Could you check a few things on this model? Use its own coordinates, in mm. A direction names the side the tool comes from. Give positions to 0.01 mm unless a question says otherwise; leave off trailing zeros. Loops run counter-clockwise (first coordinate to the right, second up) from the corner with the lowest first, then second, coordinate; pieces in that order, holes last.
1. Imagine slicing it at C-C (z = 113.65). List the corners of the cut face in (x, y) for me.
2. Thinking about a two-plate mould opening in X: for faces 3 (the cylindrical face through (42.64, 1.48, 36.93)), 4 (the flat face through (43, 1, 127)), 5 (the cylindrical face through (87.1, 1.52, 0.86)), which applies, +X half, -X half, draft (parallel to the pull), parting line (faces both ways), or undercut?
3. For faces 1 (the flat face through (43, 1, 0)), 2 (the cylindrical face through (6.03, 1.48, 48.25)), which set-ups out of +Z, -Z, +X, -X, +Y, -Y let a thin tool reach every point of the face, with its end or its side?
4. Imagine slicing it at A-A (z = 33.65). Count the separate pieces of the cut face and the enclosed holes in it, plus the area to 3 significant figures.
5. For P1, Ø4, axis at x = 44, z = 93.5, coming from the -Y side, with a flat end and sliding along its axis, tell me the tip position at first contact or that it passes through.
6. I need wall thicknesses on line 1 along X through (y, z) = (2.4, 86.5); line 2 along X through (y, z) = (0.3, 41); line 3 along X through (y, z) = (1.7, 50.5). Which ranges of each line are inside material? Lowest first, please.
7. Imagine slicing it at B-B (x = 6). List the corners of the cut face in (y, z) for me.
```python
from build123d import *

# Parameters (mm, degrees)
SKETCH_1_W      = 88
SKETCH_1_H      = 127
SKETCH_1_R      = 3.55
SKETCH_1_R_2    = 2.55
EXTRUDE_1_DEPTH = 3
FILLET_1_R      = 3


with BuildPart() as part:
    # 草图1 → 凸台-拉伸1 (new body)
    with BuildSketch(Plane(origin=(0, 0, 0), x_dir=(1, 0, 0), z_dir=(0, 1, 0))):
        with Locations((44, -63.5)):
            Rectangle(SKETCH_1_W, SKETCH_1_H)
        with Locations(Location((13.68, -13.65, 0), (0, 0, 270))):
            Circle(SKETCH_1_R, mode=Mode.SUBTRACT)
        with Locations(Location((44, -13.65, 0), (0, 0, 270))):
            Circle(SKETCH_1_R, mode=Mode.SUBTRACT)
        with Locations(Location((74.32, -13.65, 0), (0, 0, 270))):
            Circle(SKETCH_1_R, mode=Mode.SUBTRACT)
        with Locations(Location((44, -23.65, 0), (0, 0, 270))):
            Circle(SKETCH_1_R, mode=Mode.SUBTRACT)
        with Locations(Location((74.32, -23.65, 0), (0, 0, 270))):
            Circle(SKETCH_1_R, mode=Mode.SUBTRACT)
        with Locations(Location((44, -33.65, 0), (0, 0, 270))):
            Circle(SKETCH_1_R, mode=Mode.SUBTRACT)
        with Locations(Location((74.32, -33.65, 0), (0, 0, 270))):
            Circle(SKETCH_1_R, mode=Mode.SUBTRACT)
        with Locations(Location((44, -43.65, 0), (0, 0, 270))):
            Circle(SKETCH_1_R, mode=Mode.SUBTRACT)
        with Locations(Location((74.32, -43.65, 0), (0, 0, 270))):
            Circle(SKETCH_1_R, mode=Mode.SUBTRACT)
        with Locations(Location((13.68, -23.65, 0), (0, 0, 270))):
            Circle(SKETCH_1_R, mode=Mode.SUBTRACT)
        with Locations(Location((13.68, -33.65, 0), (0, 0, 270))):
            Circle(SKETCH_1_R, mode=Mode.SUBTRACT)
        with Locations(Location((13.68, -43.65, 0), (0, 0, 270))):
            Circle(SKETCH_1_R, mode=Mode.SUBTRACT)
        with Locations(Location((23.68, -13.65, 0), (0, 0, 270))):
            Circle(SKETCH_1_R_2, mode=Mode.SUBTRACT)
        with Locations(Location((64.32, -13.65, 0), (0, 0, 90))):
            Circle(SKETCH_1_R_2, mode=Mode.SUBTRACT)
        with Locations(Location((23.68, -23.65, 0), (0, 0, 270))):
            Circle(SKETCH_1_R_2, mode=Mode.SUBTRACT)
        with Locations(Location((64.32, -23.65, 0), (0, 0, 90))):
            Circle(SKETCH_1_R_2, mode=Mode.SUBTRACT)
        with Locations(Location((23.68, -33.65, 0), (0, 0, 270))):
            Circle(SKETCH_1_R_2, mode=Mode.SUBTRACT)
        with Locations(Location((64.32, -33.65, 0), (0, 0, 90))):
            Circle(SKETCH_1_R_2, mode=Mode.SUBTRACT)
        with Locations(Location((23.68, -43.65, 0), (0, 0, 270))):
            Circle(SKETCH_1_R_2, mode=Mode.SUBTRACT)
        with Locations(Location((64.32, -43.65, 0), (0, 0, 90))):
            Circle(SKETCH_1_R_2, mode=Mode.SUBTRACT)
        with Locations(Location((23.68, -53.65, 0), (0, 0, 270))):
            Circle(SKETCH_1_R_2, mode=Mode.SUBTRACT)
        with Locations(Location((64.32, -53.65, 0), (0, 0, 90))):
            Circle(SKETCH_1_R_2, mode=Mode.SUBTRACT)
        with Locations(Location((23.68, -63.65, 0), (0, 0, 270))):
            Circle(SKETCH_1_R_2, mode=Mode.SUBTRACT)
        with Locations(Location((64.32, -63.65, 0), (0, 0, 90))):
            Circle(SKETCH_1_R_2, mode=Mode.SUBTRACT)
        with Locations(Location((23.68, -73.65, 0), (0, 0, 270))):
            Circle(SKETCH_1_R_2, mode=Mode.SUBTRACT)
        with Locations(Location((64.32, -73.65, 0), (0, 0, 90))):
            Circle(SKETCH_1_R_2, mode=Mode.SUBTRACT)
        with Locations(Location((23.68, -83.65, 0), (0, 0, 270))):
            Circle(SKETCH_1_R_2, mode=Mode.SUBTRACT)
        with Locations(Location((64.32, -83.65, 0), (0, 0, 90))):
            Circle(SKETCH_1_R_2, mode=Mode.SUBTRACT)
        with Locations(Location((23.68, -93.65, 0), (0, 0, 270))):
            Circle(SKETCH_1_R_2, mode=Mode.SUBTRACT)
        with Locations(Location((64.32, -93.65, 0), (0, 0, 90))):
            Circle(SKETCH_1_R_2, mode=Mode.SUBTRACT)
        with Locations(Location((23.68, -103.65, 0), (0, 0, 270))):
            Circle(SKETCH_1_R_2, mode=Mode.SUBTRACT)
        with Locations(Location((64.32, -103.65, 0), (0, 0, 90))):
            Circle(SKETCH_1_R_2, mode=Mode.SUBTRACT)
        with Locations(Location((23.68, -113.65, 0), (0, 0, 270))):
            Circle(SKETCH_1_R_2, mode=Mode.SUBTRACT)
        with Locations(Location((64.32, -113.65, 0), (0, 0, 90))):
            Circle(SKETCH_1_R_2, mode=Mode.SUBTRACT)
        with Locations(Location((29.18, -48.68, 0), (0, 0, 270))):
            Circle(SKETCH_1_R_2, mode=Mode.SUBTRACT)
        with Locations(Location((29.18, -78.32, 0), (0, 0, 90))):
            Circle(SKETCH_1_R_2, mode=Mode.SUBTRACT)
        with Locations(Location((58.82, -48.68, 0), (0, 0, 90))):
            Circle(SKETCH_1_R_2, mode=Mode.SUBTRACT)
        with Locations(Location((58.82, -78.32, 0), (0, 0, 270))):
            Circle(SKETCH_1_R_2, mode=Mode.SUBTRACT)
        with Locations(Location((34, -63.5, 0), (0, 0, 270))):
            Circle(SKETCH_1_R_2, mode=Mode.SUBTRACT)
        with Locations(Location((54, -63.5, 0), (0, 0, 90))):
            Circle(SKETCH_1_R_2, mode=Mode.SUBTRACT)
        with Locations(Location((44, -63.5, 0), (0, 0, 270))):
            Circle(SKETCH_1_R_2, mode=Mode.SUBTRACT)
        with Locations(Location((34, -33.65, 0), (0, 0, 270))):
            Circle(SKETCH_1_R_2, mode=Mode.SUBTRACT)
        with Locations(Location((34, -43.65, 0), (0, 0, 270))):
            Circle(SKETCH_1_R_2, mode=Mode.SUBTRACT)
        with Locations(Location((54, -43.65, 0), (0, 0, 90))):
            Circle(SKETCH_1_R_2, mode=Mode.SUBTRACT)
        with Locations(Location((54, -33.65, 0), (0, 0, 90))):
            Circle(SKETCH_1_R_2, mode=Mode.SUBTRACT)
        with Locations(Location((54, -93.35, 0), (0, 0, 270))):
            Circle(SKETCH_1_R_2, mode=Mode.SUBTRACT)
        with Locations(Location((54, -83.35, 0), (0, 0, 270))):
            Circle(SKETCH_1_R_2, mode=Mode.SUBTRACT)
        with Locations(Location((34, -83.35, 0), (0, 0, 90))):
            Circle(SKETCH_1_R_2, mode=Mode.SUBTRACT)
        with Locations(Location((34, -93.35, 0), (0, 0, 90))):
            Circle(SKETCH_1_R_2, mode=Mode.SUBTRACT)
        with Locations(Location((44, -53.65, 0), (0, 0, 270))):
            Circle(SKETCH_1_R_2, mode=Mode.SUBTRACT)
        with Locations(Location((44, -73.5, 0), (0, 0, 270))):
            Circle(SKETCH_1_R_2, mode=Mode.SUBTRACT)
        with Locations(Location((44, -83.5, 0), (0, 0, 270))):
            Circle(SKETCH_1_R_2, mode=Mode.SUBTRACT)
        with Locations(Location((44, -93.5, 0), (0, 0, 270))):
            Circle(SKETCH_1_R_2, mode=Mode.SUBTRACT)
        with Locations(Location((44, -103.5, 0), (0, 0, 270))):
            Circle(SKETCH_1_R_2, mode=Mode.SUBTRACT)
        with Locations(Location((44, -113.5, 0), (0, 0, 270))):
            Circle(SKETCH_1_R_2, mode=Mode.SUBTRACT)
        with Locations(Location((13.68, -83.65, 0), (0, 0, 270))):
            Circle(SKETCH_1_R_2, mode=Mode.SUBTRACT)
        with Locations(Location((74.32, -83.65, 0), (0, 0, 90))):
            Circle(SKETCH_1_R_2, mode=Mode.SUBTRACT)
        with Locations(Location((13.68, -93.65, 0), (0, 0, 270))):
            Circle(SKETCH_1_R_2, mode=Mode.SUBTRACT)
        with Locations(Location((74.32, -93.65, 0), (0, 0, 90))):
            Circle(SKETCH_1_R_2, mode=Mode.SUBTRACT)
        with Locations(Location((13.68, -103.65, 0), (0, 0, 270))):
            Circle(SKETCH_1_R_2, mode=Mode.SUBTRACT)
        with Locations(Location((74.32, -103.65, 0), (0, 0, 90))):
            Circle(SKETCH_1_R_2, mode=Mode.SUBTRACT)
        with Locations(Location((13.68, -113.65, 0), (0, 0, 270))):
            Circle(SKETCH_1_R_2, mode=Mode.SUBTRACT)
        with Locations(Location((74.32, -113.65, 0), (0, 0, 90))):
            Circle(SKETCH_1_R_2, mode=Mode.SUBTRACT)
        with BuildLine():
            Line((7.5, -40.25), (7.5, -46.75))
            ThreePointArc((7.5, -46.75), (6, -48.25), (4.5, -46.75))
            Line((4.5, -46.75), (4.5, -40.25))
            ThreePointArc((4.5, -40.25), (6, -38.75), (7.5, -40.25))
        make_face(mode=Mode.SUBTRACT)
        with BuildLine():
            Line((7.5, -60.25), (7.5, -66.75))
            ThreePointArc((7.5, -66.75), (6, -68.25), (4.5, -66.75))
            Line((4.5, -66.75), (4.5, -60.25))
            ThreePointArc((4.5, -60.25), (6, -58.75), (7.5, -60.25))
        make_face(mode=Mode.SUBTRACT)
        with BuildLine():
            Line((7.5, -86.75), (7.5, -80.25))
            ThreePointArc((7.5, -80.25), (6, -78.75), (4.5, -80.25))
            Line((4.5, -80.25), (4.5, -86.75))
            ThreePointArc((4.5, -86.75), (6, -88.25), (7.5, -86.75))
        make_face(mode=Mode.SUBTRACT)
        with BuildLine():
            Line((80.5, -86.75), (80.5, -80.25))
            ThreePointArc((80.5, -80.25), (82, -78.75), (83.5, -80.25))
            Line((83.5, -80.25), (83.5, -86.75))
            ThreePointArc((83.5, -86.75), (82, -88.25), (80.5, -86.75))
        make_face(mode=Mode.SUBTRACT)
        with BuildLine():
            Line((80.5, -60.25), (80.5, -66.75))
            ThreePointArc((80.5, -66.75), (82, -68.25), (83.5, -66.75))
            Line((83.5, -66.75), (83.5, -60.25))
            ThreePointArc((83.5, -60.25), (82, -58.75), (80.5, -60.25))
        make_face(mode=Mode.SUBTRACT)
        with BuildLine():
            Line((80.5, -40.25), (80.5, -46.75))
            ThreePointArc((80.5, -46.75), (82, -48.25), (83.5, -46.75))
            Line((83.5, -46.75), (83.5, -40.25))
            ThreePointArc((83.5, -40.25), (82, -38.75), (80.5, -40.25))
        make_face(mode=Mode.SUBTRACT)
        with BuildLine():
            Line((16.18, -53.81), (16.18, -73.19))
            ThreePointArc((16.18, -73.19), (13.68, -75.69), (11.18, -73.19))
            Line((11.18, -73.19), (11.18, -53.81))
            ThreePointArc((11.18, -53.81), (13.68, -51.31), (16.18, -53.81))
        make_face(mode=Mode.SUBTRACT)
        with BuildLine():
            Line((71.82, -53.81), (71.82, -73.19))
            ThreePointArc((71.82, -73.19), (74.32, -75.69), (76.82, -73.19))
            Line((76.82, -73.19), (76.82, -53.81))
            ThreePointArc((76.82, -53.81), (74.32, -51.31), (71.82, -53.81))
        make_face(mode=Mode.SUBTRACT)
    extrude(amount=EXTRUDE_1_DEPTH)

    # 圆角1
    fillet_1_edges = [part.edges().sort_by_distance(p)[0] for p in [
        (0, 1.5, 0),
        (88, 1.5, 0),
        (88, 1.5, 127),
        (0, 1.5, 127),
    ]]
    fillet(fillet_1_edges, radius=FILLET_1_R)


solid = part.part
```
Derived:
1. outline: (0, 0) - (11.13, 0) - (11.13, 3) - (0, 3) - close; (16.23, 0) - (21.13, 0) - (21.13, 3) - (16.23, 3) - close; (26.23, 0) - (41.45, 0) - (41.45, 3) - (26.23, 3) - close; (46.55, 0) - (61.77, 0) - (61.77, 3) - (46.55, 3) - close; (66.87, 0) - (71.77, 0) - (71.77, 3) - (66.87, 3) - close; (76.87, 0) - (88, 0) - (88, 3) - (76.87, 3) - close
2. face 3: undercut
2. face 4: draft
2. face 5: +X half
3. face 1: -Z, +X, -X, +Y, -Y
3. face 2: +Y, -Y
4. separate pieces: 8
4. enclosed holes: 0
4. area: 139 mm2
5. P1: passes through
6. line 1: x = 0 to 4.5, 7.5 to 80.5, 83.5 to 88
6. line 2: x = 0 to 4.5, 7.5 to 11.32, 16.04 to 41.64, 46.36 to 71.96, 76.68 to 80.5, 83.5 to 88
6. line 3: x = 0 to 27.39, 30.97 to 57.03, 60.61 to 88
7. outline: (0, 0) - (3, 0) - (3, 38.75) - (0, 38.75) - close; (0, 48.25) - (3, 48.25) - (3, 58.75) - (0, 58.75) - close; (0, 68.25) - (3, 68.25) - (3, 78.75) - (0, 78.75) - close; (0, 88.25) - (3, 88.25) - (3, 127) - (0, 127) - close
